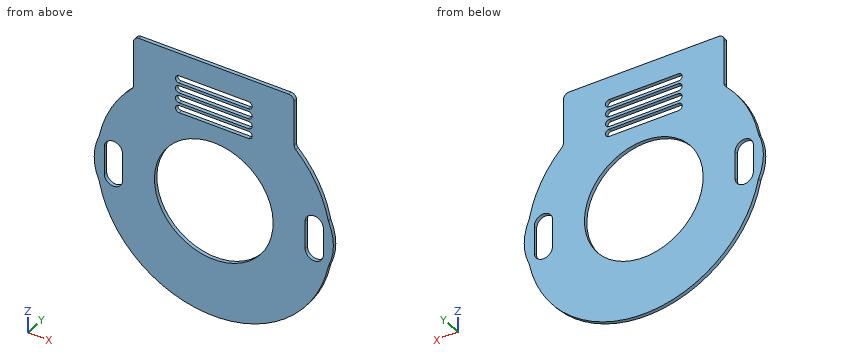
```python
from build123d import *

# Parameters (mm, degrees)
SKETCH1_R           = 32.5
BOSS_EXTRUDE1_DEPTH = 2


with BuildPart() as part:
    # Sketch1 → Boss-Extrude1 (new body)
    with BuildSketch(Plane(origin=(0, 0, 0), x_dir=(1, 0, 0), z_dir=(0, 1, 0))):
        with BuildLine():
            Line((-41, -75), (41, -75))
            ThreePointArc((41, -75), (43.121320344, -74.121320344), (44, -72))
            Line((44, -72), (44, -47.749345545))
            ThreePointArc((44, -47.749345545), (44.232922766, -46.590344431), (44.895522388, -45.611315148))
            ThreePointArc((44.895522388, -45.611315148), (56.240897341, -30.544417924), (62.701869476, -12.824802695))
            ThreePointArc((62.701869476, -12.824802695), (62.784364017, -12.509712717), (62.900531241, -12.20542302))
            ThreePointArc((62.900531241, -12.20542302), (65.495647572, 0), (62.900531241, 12.20542302))
            ThreePointArc((62.900531241, 12.20542302), (62.784364017, 12.509712717), (62.701869476, 12.824802695))
            ThreePointArc((62.701869476, 12.824802695), (0, 64), (-62.701869476, 12.824802695))
            ThreePointArc((-62.701869476, 12.824802695), (-62.784364017, 12.509712717), (-62.900531241, 12.20542302))
            ThreePointArc((-62.900531241, 12.20542302), (-65.495647572, 0), (-62.900531241, -12.20542302))
            ThreePointArc((-62.900531241, -12.20542302), (-62.784364017, -12.509712717), (-62.701869476, -12.824802695))
            ThreePointArc((-62.701869476, -12.824802695), (-56.240897341, -30.544417924), (-44.895522388, -45.611315148))
            ThreePointArc((-44.895522388, -45.611315148), (-44.232922766, -46.590344431), (-44, -47.749345545))
            Line((-44, -47.749345545), (-44, -72))
            ThreePointArc((-44, -72), (-43.121320344, -74.121320344), (-41, -75))
        make_face()
        with Locations(Location((0, 0, 0), (0, 0, 270))):
            Circle(SKETCH1_R, mode=Mode.SUBTRACT)
        with BuildLine():
            Line((-50, 7.5), (-50, -7.5))
            ThreePointArc((-50, -7.5), (-55, -12.5), (-60, -7.5))
            Line((-60, -7.5), (-60, 7.5))
            ThreePointArc((-60, 7.5), (-55, 12.5), (-50, 7.5))
        make_face(mode=Mode.SUBTRACT)
        with BuildLine():
            Line((50, 7.5), (50, -7.5))
            ThreePointArc((50, -7.5), (55, -12.5), (60, -7.5))
            Line((60, -7.5), (60, 7.5))
            ThreePointArc((60, 7.5), (55, 12.5), (50, 7.5))
        make_face(mode=Mode.SUBTRACT)
        with BuildLine():
            Line((-19, -42), (19, -42))
            ThreePointArc((19, -42), (21, -44), (19, -46))
            Line((19, -46), (-19, -46))
            ThreePointArc((-19, -46), (-21, -44), (-19, -42))
        make_face(mode=Mode.SUBTRACT)
        with BuildLine():
            Line((-19, -47.5), (19, -47.5))
            ThreePointArc((19, -47.5), (21, -49.5), (19, -51.5))
            Line((19, -51.5), (-19, -51.5))
            ThreePointArc((-19, -51.5), (-21, -49.5), (-19, -47.5))
        make_face(mode=Mode.SUBTRACT)
        with BuildLine():
            Line((-19, -53), (19, -53))
            ThreePointArc((19, -53), (21, -55), (19, -57))
            Line((19, -57), (-19, -57))
            ThreePointArc((-19, -57), (-21, -55), (-19, -53))
        make_face(mode=Mode.SUBTRACT)
        with BuildLine():
            Line((-19, -58.5), (19, -58.5))
            ThreePointArc((19, -58.5), (21, -60.5), (19, -62.5))
            Line((19, -62.5), (-19, -62.5))
            ThreePointArc((-19, -62.5), (-21, -60.5), (-19, -58.5))
        make_face(mode=Mode.SUBTRACT)
    extrude(amount=BOSS_EXTRUDE1_DEPTH)


solid = part.part
```
For this review, take the finished solid that the model builds, in its own axes (mm). Round coordinates to 2 decimals unless told otherwise and drop trailing zeros. Write each loop counter-clockwise with the first axis right and the second up, starting at its lowest first coordinate (ties: lowest second). Pieces come first, ordered by that corner, then holes. Notation, with made-up numbers: (-15.5, -30) - (21.5, -30) arc R24 ccw to (21.5, -12) - close; hole circle Ø1 at (-37.5, 73). An arc over 180 degrees is marked (long way). Write each question's results on one line, items separated by ' | '.
Item 1: Take a section at A-A on x = 0. State the section outline as (y, z) points.
Calculated:
outline: (0, -64) - (2, -64) - (2, -32.5) - (0, -32.5) - close; (0, 32.5) - (2, 32.5) - (2, 42) - (0, 42) - close; (0, 46) - (2, 46) - (2, 47.5) - (0, 47.5) - close; (0, 51.5) - (2, 51.5) - (2, 53) - (0, 53) - close; (0, 57) - (2, 57) - (2, 58.5) - (0, 58.5) - close; (0, 62.5) - (2, 62.5) - (2, 75) - (0, 75) - close
Item 2: To check wall thickness, follow line 1 along Z through (x, y) = (-5, 1.1); line 2 along X through (y, z) = (0.75, -10); line 3 along Z through (x, y) = (9.5, 0.45). State the ranges of each line that lie inside material, in increasing order. Write a range as from..to.
Calculated:
line 1: z = -63.8..-32.11, 32.11..42, 46..47.5, 51.5..53, 57..58.5, 62.5..75 | line 2: x = -63.78..-59.33, -50.67..-30.92, 30.92..50.67, 59.33..63.78 | line 3: z = -63.29..-31.08, 31.08..42, 46..47.5, 51.5..53, 57..58.5, 62.5..75
Item 3: Take a section at B-B on z = 17.5. State the section outline as (x, y) points, then the cut area to 3 significant figures.
Calculated:
outline: (-61.56, 0) - (-27.39, 0) - (-27.39, 2) - (-61.56, 2) - close; (27.39, 0) - (61.56, 0) - (61.56, 2) - (27.39, 2) - close | area: 137 mm^2
Item 4: For pin 1 (0.6 mm diameter, centred on x = -9, y = 1.5, fed in from -Z); pin 2 (0.6 mm diameter, centred on y = 0.5, z = 54.5, fed in from +X); pin 3 (1 mm diameter, centred on y = 1, z = -3, fed in from -X), all flat-tipped, find the tip position at first contact; note any pin that passes through.
Calculated:
pin 1: stops at z = -63.41 | pin 2: stops at x = 44 | pin 3: stops at x = -65.39
Item 5: Take a section at D-D on y = 0.85. Count the separate pieces of the cut face and the enclosed holes in it, then the cut area to 3 significant figures.
Calculated:
separate pieces: 1 | enclosed holes: 7 | area: 9,930 mm^2
Item 6: Take a section at C-C on x = 55. State the section outline as (y, z) points.
Calculated:
outline: (0, -32.73) - (2, -32.73) - (2, -12.5) - (0, -12.5) - close; (0, 12.5) - (2, 12.5) - (2, 32.73) - (0, 32.73) - close
